```python
from build123d import *

# Parameters (mm, degrees)
F0_W      = 7.6
F0_H      = 6
F1_DEPTH  = 30
F2_W      = 10.2
F2_H      = 1.2
F2_W_2    = 7.35
F2_W_3    = 10.05
F2_W_4    = 1.2
F3_DEPTH  = 10
F4_W      = 3.1
F4_H      = 6
F4_W_2    = 3.15
F5_DEPTH  = 25
F4_W_3    = 7.35
F6_DEPTH  = 3
F2_H_2    = 10
F7_DEPTH  = 30.8
F8_DEPTH  = 25
F9_W      = 8.2
F9_H      = 8.16
F10_DEPTH = 25
F12_DEPTH = 25
F14_DEPTH = 25
F15_DEPTH = 1.2


with BuildPart() as f1:
    # F0 (on Right) → F1 (new body)
    with BuildSketch(Plane.YZ):
        Polygon((-18.5999230509, 30.0000671301), (-19.9999230509, 30.0000671301), (-19.9999230509, 24.0000671301), (-9.9999230509, 6.0000671301), (-9.9999230509, 6.71301e-05), (-8.7999230509, 6.71301e-05), (-8.7999230509, 6.0000671301), (-18.5999230509, 24.0000671301), align=None)
        Polygon((-11.2499230509, 24.0000671301), (-18.5999230509, 24.0000671301), (-8.7999230509, 6.0000671301), (-1.1999230509, 6.0000671301), align=None)
        Polygon((-9.9999230509, 30.0000671301), (-11.2499230509, 30.0000671301), (-11.2499230509, 24.0000671301), (-1.1999230509, 6.0000671301), (-1.1999230509, 6.71301e-05), (7.69491e-05, 6.71301e-05), (7.69491e-05, 6.0000671301), (-9.9999230509, 24.0000671301), align=None)
        with Locations((-4.9999230509, 3.0000671301)):
            Rectangle(F0_W, F0_H)
    extrude(amount=F1_DEPTH)

    # F2 (on face) → F3 (join)
    with BuildSketch(Plane(origin=(0, 0, 6.71301e-05), x_dir=(1, 0, 0), z_dir=(0, 0, -1))):
        with Locations((5.1, 10.5999230509)):
            Rectangle(F2_W, F2_H)
        with Locations((15.075, 10.5999230509)):
            Rectangle(F2_W_2, F2_H)
        with Locations((24.975, 10.5999230509)):
            Rectangle(F2_W_3, F2_H)
        with Locations((10.8, 10.5999230509)):
            Rectangle(F2_W_4, F2_H)
        with Locations((19.35, 10.5999230509)):
            Rectangle(F2_W_4, F2_H)
    extrude(amount=-F3_DEPTH)

    # F4 (on face) → F5 (join)
    with BuildSketch(Plane(origin=(0, -9.9999230509, 0), x_dir=(-1, 0, 0), z_dir=(0, 1, 0))):
        with Locations((-20.25, 27.0000671301)):
            Rectangle(F4_W, F4_H)
        with Locations((-9.775, 27.0000671301)):
            Rectangle(F4_W_2, F4_H)
    extrude(amount=F5_DEPTH)

    # F4 (on face) → F6 (cut)
    with BuildSketch(Plane(origin=(0, -9.9999230509, 0), x_dir=(-1, 0, 0), z_dir=(0, 1, 0))):
        with Locations((-15.025, 27.0000671301)):
            Rectangle(F4_W_3, F4_H)
    extrude(amount=-F6_DEPTH, mode=Mode.SUBTRACT)

    # F2 (on face) → F7 (cut)
    with BuildSketch(Plane(origin=(0, 0, 6.71301e-05), x_dir=(1, 0, 0), z_dir=(0, 0, -1))):
        with Locations((15.075, 4.9999230509)):
            Rectangle(F2_W_2, F2_H_2)
    extrude(amount=-F7_DEPTH, mode=Mode.SUBTRACT)

    # F0 (on Right) → F8 (cut)
    with BuildSketch(Plane.YZ):
        Polygon((7.69491e-05, 51.0639390725), (7.69491e-05, 30.0000671301), (7.69491e-05, 6.0000671301), (43.8302202369, 6.0000671301), (43.8302202369, 51.0639390725), align=None)
    extrude(amount=F8_DEPTH, mode=Mode.SUBTRACT)

    # F9 (on face) → F10 (cut)
    with BuildSketch(Plane.XZ.offset(11.1999230509)):
        with Locations((4.1, 4.0800671301)):
            Rectangle(F9_W, F9_H)
        with Locations((25.9, 4.0800671301)):
            Rectangle(F9_W, F9_H)
    extrude(amount=-F10_DEPTH, mode=Mode.SUBTRACT)

    # F11 (on Front) → F12 (cut)
    with BuildSketch(Plane.XZ):
        Polygon((0, 24), (0, 8.16), (8.2, 8.16), align=None)
        Polygon((30, 24), (21.8, 8.16), (30, 8.16), align=None)
    extrude(amount=F12_DEPTH, mode=Mode.SUBTRACT)

    # F13 (on face) → F14 (cut)
    with BuildSketch(Plane(origin=(0, -18.5999230509, 0), x_dir=(-1, 0, 0), z_dir=(0, 1, 0))):
        with BuildLine():
            ThreePointArc((-17.5, 30.0000671301), (-17.466917068, 29.5947028748), (-17.3685438565, 29.2000671301))
            ThreePointArc((-17.3685438565, 29.2000671301), (-14.5946357448, 27.533150062), (-12.5, 30.0000671301))
            Line((-12.5, 30.0000671301), (-17.5, 30.0000671301))
        make_face()
    extrude(amount=-F14_DEPTH, mode=Mode.SUBTRACT)

    # F13 (on face) → F15 (join)
    with BuildSketch(Plane(origin=(0, -18.5999230509, 0), x_dir=(-1, 0, 0), z_dir=(0, 1, 0))):
        with BuildLine():
            ThreePointArc((-11.5, 30.0000671301), (-15.4026738592, 33.4768262191), (-18.4073450075, 29.2000671301))
            ThreePointArc((-18.4073450075, 29.2000671301), (-14.5973261408, 26.523308041), (-11.5, 30.0000671301))
        make_face()
        with BuildLine():
            ThreePointArc((-12.5, 30.0000671301), (-14.5946357448, 27.533150062), (-17.3685438565, 29.2000671301))
            ThreePointArc((-17.3685438565, 29.2000671301), (-15.4053642552, 32.4669841981), (-12.5, 30.0000671301))
        make_face(mode=Mode.SUBTRACT)
    extrude(amount=-F15_DEPTH)


solid = f1.part
```
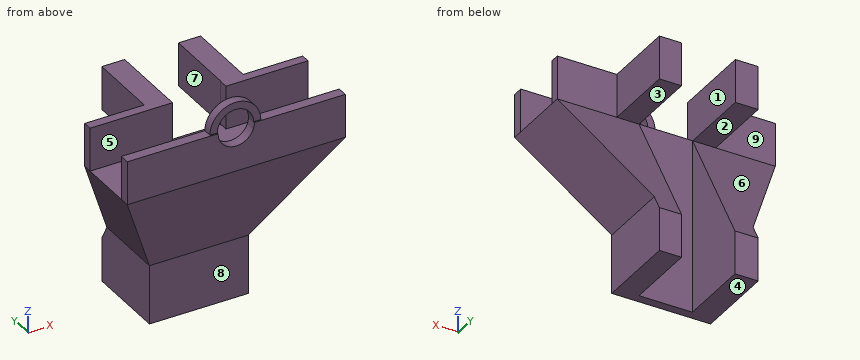
Could you check a few things on this model? Use its own coordinates, in mm. Face numbers are marked on the shaded views. A direction names the side the tool comes from. Round coordinates to 2 decimals unless told otherwise and drop trailing zeros. Write each loop counter-clockwise with the first axis right and the second up, starting at its lowest first coordinate (ties: lowest second). Pieces come first, ordered by that corner, then holes. Notation, with made-up numbers: M -13.5,33 L 23.5,33 A11 cw 23.5,48 Z; hole C 4.5,-25 d3. An arc over 180 degrees is marked long. Answer in a Markdown table with one row per item. Add a question column.
Q1. Imagine slicing it at D-D (z = 3.5). Please give me the cut outline in (x, y).
Q2. On a 3-axis mill with a long thin cutter (end or side, diameter ignored), from which of +Z, -Z, +X, -X, +Y, -Y can I reach the whole of each face in a straight line? I mean the marked faces 5, 6, 7, 8 and 9. Say none if no direction works.
Q3. If I drill on line 1 (Y direction, x = 28, z = 27); line 2 (X direction, y = -4, z = 5); line 3 (Y direction, x = 16, z = 5), over which ranges is the centre line in solid material (lowest first)? Write a range as from..to.
Q4. If we mould it in two halves opening along Z, with no side actions, what happens to the marked faces 1, 2, 3 and 4? For each: +Z half, -Z half, draft (parallel to the pull), parting line (faces both ways), or undercut.
Q5. Imagine slicing it at B-B (z = 25). Please give me the cut outline in (x, y).
Q6. Imagine slicing it at A-A (x = 15). Please give me the cut outline in (y, z), then the cut area to 3 significant figures.
Q7. Imagine slicing it at C-C (y = -5.5). Give the number of separate pieces and of enclosed holes in the cut face, then the cut area to 3 significant figures.
Q8. Will these pins go through, and if not, where does the flat tip stop? pin 1 Ø5 at (y, z) = (-4.5, 25.5) entering from -X; pin 2 Ø3 at (x, z) = (15.5, 8.5) entering from -Y; pin 3 Ø4 at (x, y) = (27, -8.5) entering from -Z; pin 4 Ø1.5 at (x, y) = (17.5, -6.5) entering from -Z.
Values:
| question | item | result |
|---|---|---|
| 1 | outline | M 8.2,-11.2 L 21.8,-11.2 L 21.8,0 L 18.75,0 L 18.75,-10 L 11.4,-10 L 11.4,0 L 8.2,0 Z |
| 2 | face 5 | +Z, +X, -X |
| 2 | face 6 | +X, -X, +Y |
| 2 | face 7 | +Z, -Z, +Y |
| 2 | face 8 | -Z, +X, -X, -Y |
| 2 | face 9 | +Z, -X, +Y |
| 3 | line 1 | -20..-18.6, -11.25..-10 |
| 3 | line 2 | 8.2..11.4, 18.75..21.8 |
| 3 | line 3 | -11.2..-10 |
| 4 | face 1 | draft |
| 4 | face 2 | undercut |
| 4 | face 3 | undercut |
| 4 | face 4 | -Z half |
| 5 | outline | M 0,-20 L 30,-20 L 30,-18.6 L 0,-18.6 Z; M 0,-11.25 L 11.35,-11.25 L 11.35,0 L 8.2,0 L 8.2,-10 L 0,-10 Z; M 18.7,-11.25 L 30,-11.25 L 30,-10 L 21.8,-10 L 21.8,0 L 18.75,0 L 18.75,-10 L 18.7,-10 Z |
| 6 | outline | M -20,24 L -11.2,8.16 L -11.2,0 L -10,0 L -10,24 L -18.6,24 L -18.6,27.5 L -20,27.5 Z; M -19.8,32.5 L -18.6,32.5 L -18.6,33.5 L -19.8,33.5 Z |
| 6 | area | 105 mm^2 |
| 7 | separate pieces | 4 |
| 7 | enclosed holes | 0 |
| 7 | area | 168 mm^2 |
| 8 | pin 1 | x = 8.2 |
| 8 | pin 2 | y = -12.22 |
| 8 | pin 3 | z = 14.34 |
| 8 | pin 4 | through |
